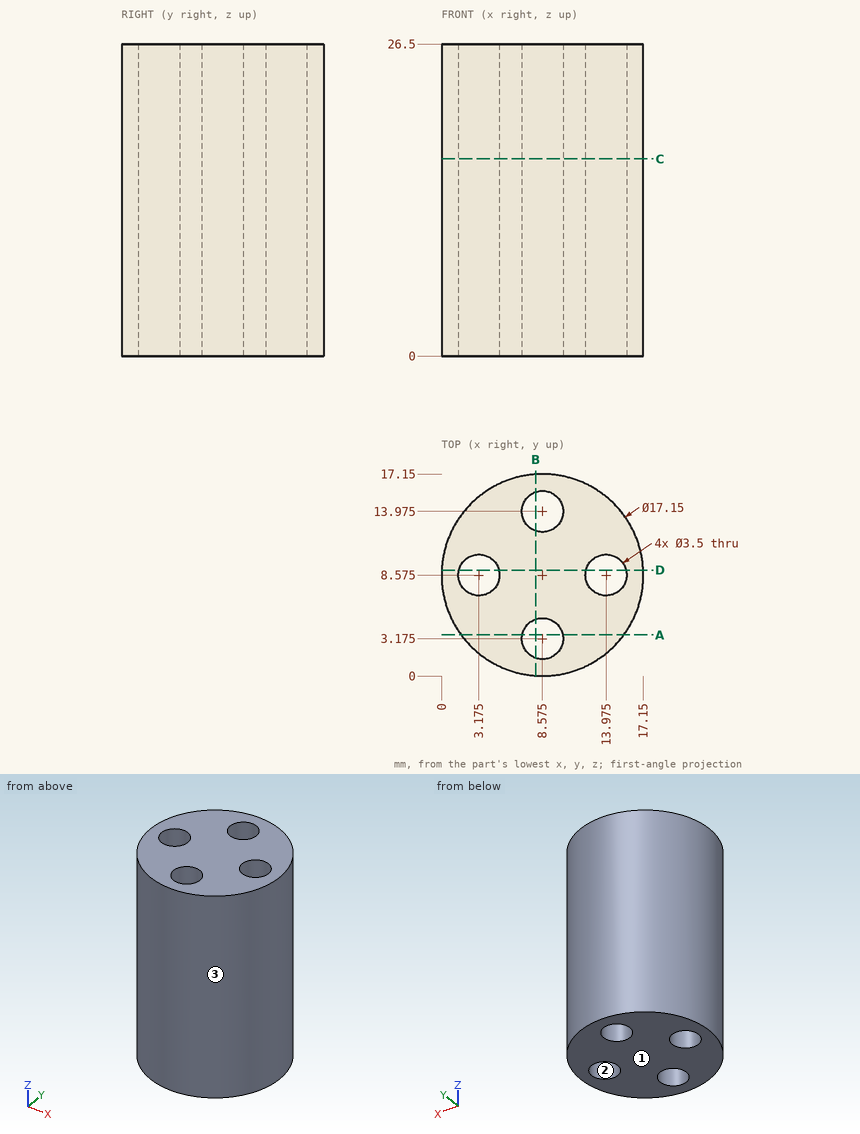
Can you work these out from the drawing? Everything is in mm from the part's minimum corner. Round coordinates to 2 decimals unless told otherwise and drop trailing zeros. Write each loop counter-clockwise with the first axis right and the second up, starting at its lowest first coordinate (ties: lowest second). Pieces come first, ordered by that corner, then holes. Notation, with made-up numbers: (-9, 19.5) - (27, 19.5) arc R10 cw to (27, 38.5) - close; hole circle Ø8 at (-34.75, 73). An arc over 180 degrees is marked (long way). Put each result on its own line as item: value. Start each with the question number.
(1) Thinking about a two-plate mould opening in Y: for the marked faces 1, 2 and 3, which applies, released by +Y, released by -Y, zero draft, split by the parting line, or undercut?
(2) Will these pins go through, and if not, where does the flat tip stop? pin 1 (4 mm diameter, centred on y = 3, z = 18.5, fed in from +X); pin 2 (2 mm diameter, centred on x = 10, z = 17.5, fed in from -Y); pin 3 (5 mm diameter, centred on y = 13.5, z = 19.5, fed in from -X).
(3) I want a section at D-D, the plane y = 9. Please give me the cut outline in (x, z), plus the area to 3 significant figures.
(4) I want a section at C-C, the plane z = 16.75. Please give me the cut outline in (x, y) (3 decimals).
(5) I need wall thicknesses on probe 1 along X at (y, z) = (8.5, 23.75); probe 2 along Y at (x, z) = (9.5, 6); probe 3 along Y at (x, z) = (7.5, 14). Which ranges of each line are inside material? Lowest first, please.
(6) I want a section at A-A, the plane y = 3.5. Please give me the cut outline in (x, z), plus the area to 3 significant figures.
(7) I want a section at B-B, the plane x = 8. Please give me the cut outline in (y, z).
Here are the results:
1. face 1: zero draft
1. face 2: undercut
1. face 3: split by the parting line
2. pin 1: stops at x = 16.37
2. pin 2: stops at y = 0.01
2. pin 3: stops at x = 0.35
3. outline: (0.01, 0) - (1.48, 0) - (1.48, 26.5) - (0.01, 26.5) - close; (4.87, 0) - (12.28, 0) - (12.28, 26.5) - (4.87, 26.5) - close; (15.67, 0) - (17.14, 0) - (17.14, 26.5) - (15.67, 26.5) - close
3. area: 274 mm^2
4. outline: circle Ø17.15 at (8.575, 8.575); hole circle Ø3.5 at (3.175, 8.575); hole circle Ø3.5 at (8.575, 3.175); hole circle Ø3.5 at (8.575, 13.975); hole circle Ø3.5 at (13.975, 8.575)
5. probe 1: x = 0 to 1.43, 4.92 to 12.23, 15.72 to 17.15
5. probe 2: y = 0.05 to 1.69, 4.66 to 12.49, 15.46 to 17.1
5. probe 3: y = 0.07 to 1.79, 4.56 to 12.59, 15.36 to 17.08
6. outline: (1.66, 0) - (6.86, 0) - (6.86, 26.5) - (1.66, 26.5) - close; (10.29, 0) - (15.49, 0) - (15.49, 26.5) - (10.29, 26.5) - close
6. area: 275 mm^2
7. outline: (0.02, 0) - (1.52, 0) - (1.52, 26.5) - (0.02, 26.5) - close; (4.83, 0) - (12.32, 0) - (12.32, 26.5) - (4.83, 26.5) - close; (15.63, 0) - (17.13, 0) - (17.13, 26.5) - (15.63, 26.5) - close
